```python
from build123d import *

# Parameters (mm, degrees)
SKETCH_1_R            = 11
EXTRUDE_1_DEPTH       = 10
CUT_EXTRUDE_1_DEPTH   = 38.37729926
FILLET_1_R            = 1.5
M4X0_71_D             = 3.3
M4X0_71_DEPTH         = 5
M4X0_71_TIP           = 0.991420021
HOLE_WIZARD_M41_D     = 4.5
HOLE_WIZARD_M41_DEPTH = 3
M4X0_72_D             = 3.3
M4X0_72_DEPTH         = 10
M4X0_72_TIP           = 0.991420021
FILLET_2_R            = 3


with BuildPart() as part:
    # Эскиз1 → Бобышка-Вытянуть1 (new body)
    with BuildSketch(Plane.XY):
        with BuildLine():
            Line((-31.75, -12), (-9.910576673, 9.888400781))
            ThreePointArc((-9.910576673, 9.888400781), (0, 14), (9.910576673, 9.888400781))
            Line((9.910576673, 9.888400781), (31.75, -12))
            Line((31.75, -12), (31.75, -17))
            Line((31.75, -17), (-31.75, -17))
            Line((-31.75, -17), (-31.75, -12))
        make_face()
        Circle(SKETCH_1_R, mode=Mode.SUBTRACT)
    extrude(amount=EXTRUDE_1_DEPTH)

    # Эскиз2 → Вырез-Вытянуть1 (cut, through all)
    with BuildSketch(Plane.XY.offset(10)):
        Polygon((7.786881672, 7.769457757), (24.518816114, -9), (31.75, -9), (31.75, -12), (23.274206636, -12), (10.995743008, 0.305999515), align=None)
    extrude(amount=-CUT_EXTRUDE_1_DEPTH, mode=Mode.SUBTRACT)

    # Скругление1
    fillet_1_edges = [part.edges().sort_by_distance(p)[0] for p in [
        (23.274206636, -12, 5),
        (24.518816114, -9, 5),
        (28.756712796, -9, 5),
        (10.995743008, 0.305999515, 5),
    ]]
    fillet(fillet_1_edges, radius=FILLET_1_R - 0.0001)  # a hair under: the kernel refuses the full size

    # Отверстие обработанное метчиком M4x0.71
    with Locations(Plane(origin=(0, -17, 0), x_dir=(-1, 0, 0), z_dir=(0, -1, 0))):
        with Locations((26.75, -5), (-26.75, -5)):
            Hole(M4X0_71_D / 2, depth=M4X0_71_DEPTH)
            with Locations((0, 0, -(M4X0_71_DEPTH + M4X0_71_TIP / 2))):  # 118° drill point
                Cone(0, M4X0_71_D / 2, M4X0_71_TIP, mode=Mode.SUBTRACT)

    # Отверстие с зазором M41
    with Locations(Plane(origin=(9.910576673, 9.888400781, 0), x_dir=(0, 0, -1), z_dir=(0.7078983337955254, 0.7063143415006656, 0))):
        with Locations((-5, -16.066771723)):
            Hole(HOLE_WIZARD_M41_D / 2, depth=HOLE_WIZARD_M41_DEPTH)

    # Отверстие обработанное метчиком M4x0.72
    with Locations(Plane(origin=(5.66318667, 5.650514732, 0), x_dir=(0, 0, -1), z_dir=(0.7078983337955258, 0.7063143415006653, 0))):
        with Locations((-5, -16.066771723)):
            Hole(M4X0_72_D / 2, depth=M4X0_72_DEPTH)
            with Locations((0, 0, -(M4X0_72_DEPTH + M4X0_72_TIP / 2))):  # 118° drill point
                Cone(0, M4X0_72_D / 2, M4X0_72_TIP, mode=Mode.SUBTRACT)

    # Скругление2
    fillet_2_edges = [part.edges().sort_by_distance(p)[0] for p in [
        (-31.75, -12, 5),
        (31.75, -12, 5),
    ]]
    fillet(fillet_2_edges, radius=FILLET_2_R)


solid = part.part
```
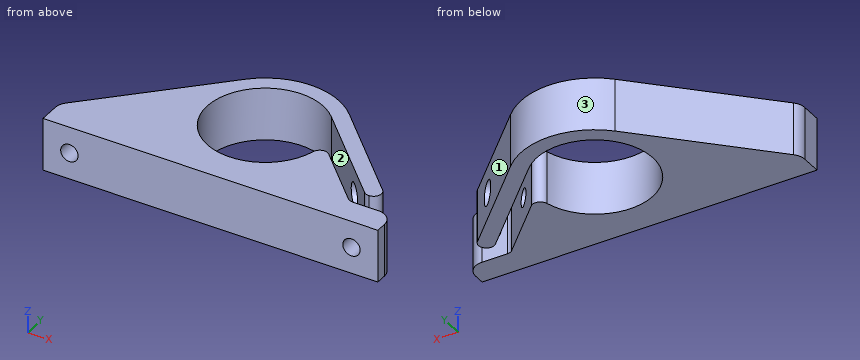
Model file for the job. Use its own axes, mm. Face numbers are marked on the shaded views. Give positions to 0.01 mm unless a question says otherwise; leave off trailing zeros. Loops run counter-clockwise (first coordinate to the right, second up) from the corner with the lowest first, then second, coordinate; pieces in that order, holes last. Notation, with made-up numbers: (26.5, 70) -> (52.5, 70) arc R25 ccw to (52.5, 109) -> close; hole circle Ø6 at (-2, 5.25). An arc over 180 degrees is marked (long way). Use CSV: the item, a comma, the result in double quotes. Start each with the question number.
1) Flat gauge pins, fed straight in: pin 1 Ø5.5 at (x, z) = (26.75, 5) entering from +Y; pin 2 Ø4 at (x, z) = (-21, 1.5) entering from +Y; pin 3 Ø6 at (x, y) = (6.5, -8.5) entering from -Z; pin 4 Ø2.5 at (x, z) = (-26.75, 5) entering from -Y. Where does each tip first touch, or does it go through?
2) Slice it at D-D on x = -12. Give the cut face in (y, z), plus the area to 3 significant figures.
3) Mould opens along X. For the marked faces 1, 2 and 3 say: released by +X, released by -X, zero draft, split by the parting line, or undercut.
4) Slice it at A-A on x = 0. Give the cut face in (y, z).
5) Slice it at C-C on x = 15. Give the number of separate pieces and of enclosed holes in the cut face, plus the area to 3 significant figures.
6) Wall check: line 1 (X direction, y = -15.45, z = 5); line 2 (X direction, y = -13, z = 5); line 3 (X direction, y = -6.5, z = 7.5). Give the ranges that are in metal, low to high.
Computed values:
1,pin 1,"stops at y = -4.23"
1,pin 2,"stops at y = 0.78"
1,pin 3,"stops at z = 0"
1,pin 4,"stops at y = -11.76"
2,outline,"(-17, 0) -> (7.79, 0) -> (7.79, 10) -> (-17, 10) -> close"
2,area,"248 mm^2"
3,face 1,"released by +X"
3,face 2,"undercut"
3,face 3,"split by the parting line"
4,outline,"(-17, 0) -> (-11, 0) -> (-11, 10) -> (-17, 10) -> close; (11, 0) -> (14, 0) -> (14, 10) -> (11, 10) -> close"
5,separate pieces,"2"
5,enclosed holes,"1"
5,area,"163 mm^2"
6,line 1,"x = -31.75 to -28.4, -25.1 to 25.1, 28.4 to 31.75"
6,line 2,"x = -31.74 to -28.4, -25.1 to 9.11, 12.05 to 25.1, 28.4 to 30.99"
6,line 3,"x = -26.26 to -8.87, 8.87 to 17.79, 22.02 to 26.26"
